Autodesk Inventor part; units mm, degrees
ref_plane "YZ Plane" through (0, 0, 0) normal (1, 0, 0) x (0, 1, 0)
ref_plane "XZ Plane" through (0, 0, 0) normal (0, 1, 0) x (-1, 0, 0)
ref_plane "XY Plane" through (0, 0, 0) normal (0, 0, 1) x (1, 0, 0)
ref_plane "Work Plane3" through (-98.2192, 25.6748, -72.651) normal (0, 1, 0) x (1, 0, 0)
sketch "Sketch1" plane through (-98.2192, 25.6748, -72.651) normal (0, 1, 0) x (1, 0, 0)
  line L0 (108.2722, -112.7231) -> (109.1382, -112.2231) construction
  line L1 (108.6382, -111.3571) -> (109.1382, -112.2231) construction
  line L2 (101.5917, -99.1522) -> (114.8917, -122.1885)
  line L3 (114.8917, -122.1885) -> (108.6563, -125.7885)
  line L4 (108.6563, -125.7885) -> (109.9613, -128.0488)
  line L5 (109.9613, -128.0488) -> (107.3632, -129.5488)
  line L6 (107.3632, -129.5488) -> (106.3632, -127.8168)
  line L7 (106.3632, -127.8168) -> (98.8635, -132.1468)
  line L8 (98.8635, -132.1468) -> (103.1935, -139.6466)
  line L9 (79.4712, -121.2385) -> (82.4842, -126.4571) construction
  line L10 (103.1935, -139.6466) -> (98.8633, -142.1466)
  line L11 (83.0235, -104.7111) -> (90.5232, -100.3811)
  line L12 (90.5232, -100.3811) -> (88.3182, -96.5619)
  line L13 (88.3182, -96.5619) -> (90.8427, -95.1044)
  line L14 (83.0235, -104.7111) -> (78.6935, -97.2113)
  line L15 (73.6327, -111.1259) -> (88.2377, -136.4225)
  line L16 (78.6935, -97.2113) -> (74.3633, -99.7113)
  line L17 (90.8427, -95.1044) -> (85.0892, -72.651)
  line L18 (104.7842, -84.0219) -> (98.2192, -72.651)
  line L19 (98.2192, -72.651) -> (85.0892, -72.651)
  line L20 (88.2377, -136.4225) -> (98.8633, -142.1466)
  line L21 (74.3633, -99.7113) -> (73.6327, -111.1259)
  line L22 (98.2192, -72.651) -> (104.7842, -84.0219)
  line L23 (104.7842, -84.0219) -> (101.5917, -99.1522)
  dimension "d1" = 26.6
  dimension "d4" = 7.2
  dimension "d5" = 2.61
  dimension "d6" = 3
  dimension "d7" = 2
  dimension "d8" = 8.66
  dimension "d9" = 8.66
  dimension "d10" = 5
  dimension "d11" = 8.66
  dimension "d12" = 31.68
  dimension "d13" = 4.41
  dimension "d14" = 2.915
  dimension "d17" = 8.66
  dimension "d18" = 29.21
  dimension "d20" = 10.27
  dimension "d21" = 5
  dimension "d22" = 23.1789
  dimension "d23" = 13.13
  dimension "d31" = 13.13
extrude "Extrusion1" add sketch "Sketch1" along normal blind 8.66
pattern_circular "Circular Pattern2" count 3 over 360 about axis through (0, 25.6748, 0) along (0, 1, 0) of "Extrusion1"
sketch "Sketch2" plane through (-98.2192, 34.3348, -72.651) normal (0, 1, 0) x (1, 0, 0)
  line L0 (46.9822, -62.321) -> (73.5822, -62.321)
  line L1 (114.8917, -122.1885) -> (101.5917, -99.1522)
  circle A0 centre (98.2192, -72.651) radius 1.5
  line L2 (98.2192, -72.651) -> (104.7842, -84.0219) construction
  line L3 (98.2192, -72.651) -> (85.0892, -72.651) construction
  line L4 (98.2192, -72.651) -> (104.7842, -61.28) construction
  circle A1 centre (98.2192, -72.651) radius 7 construction
  circle A2 centre (101.7192, -78.7131) radius 1.5
  circle A3 centre (101.7192, -66.5888) radius 1.5
  circle A4 centre (91.2192, -72.651) radius 1.5
  dimension "d35" = 3
  dimension "d36" = 14
  dimension "d37" = 3
  dimension "d38" = 3
  dimension "d39" = 3
extrude "Extrusion2" cut sketch "Sketch2" against normal blind 10
The listing builds one solid part. Answer for the finished solid, in the listing's coordinates (mm). A direction names the side the tool comes from. Round coordinates to 2 decimals unless told otherwise and drop trailing zeros. Loops run counter-clockwise (first coordinate to the right, second up) from the corner with the lowest first, then second, coordinate; pieces in that order, holes last. Notation, with made-up numbers: (81.5, 39.25) - (128.5, 39.25) arc R22 cw to (128.5, 59.25) - close; hole circle Ø6 at (-27, 17.25). An arc over 180 degrees is marked (long way). Use one line per item in the form item = value. Start each with the question number.
1. The part is cut by section C-C on y = 32.75. Give the number of separate pieces and of enclosed holes in the cut face, then the cut area to 3 significant figures.
2. A tool of negligible diameter and unlimited length cuts with its end or side. For faces 1 (the face through (-16.2, 29.944, -37.316)), 2 (the face through (-8.78, 29.94, 25.85)), 3 (the face through (-2, 34.335, -1)), 4 (the face through (-38, 30, -10.33)), from which of +Z, -Z, +X, -X, +Y, -Y can it reach the whole face along a straight path? Write none if from no direction.
3. Consider line 1 (Z direction, x = -20, y = 26.5); line 2 (X direction, y = 29.75, z = 0); line 3 (Z direction, x = -15, y = 28.75). Determine where each line is inside the solid, lowest interval first. Write a range as [from, to].
4. The part is cut by section A-A on x = -45. Determine the outline of the cut face in (y, z).
5. The part is cut by section B-B on z = 45. Determine the outline of the cut face in (x, y), then the cut area to 3 significant figures.
6. Given pin 1 Ø3 at (y, z) = (31.5, -21.5) entering from -X; pin 2 Ø4 at (y, z) = (32.5, 31) entering from -X; pin 3 Ø3 at (y, z) = (28.5, -7) entering from +X; pin 4 Ø4 at (x, z) = (0, 0) entering from +Y, each flat-ended and moving along its own axis, determine where each tip first touches the part or whether it passes through.
7. For a pull along X with two mould halves and no side action, classify faces 5 (the face through (-1.5, 30.07, -0.07)), 6 (the face through (13.6, 29.94, 51.31)), 7 (the face through (-10.213, 29.944, 11.384)) as pulls with the +X half, pulls with the -X half, needs draft (parallel to the pull), parting line crosses it, or undercut.
Geometry check:
q1.separate_pieces = 1
q1.enclosed_holes = 4
q1.area = 4,340 mm^2
q2.face_1 = -Z, +Y, -Y
q2.face_2 = +Y, -Y
q2.face_3 = +Z, -Z, +X, -X, +Y
q2.face_4 = +Z, -X, +Y, -Y
q3.line_1 = [-39.85, -29.19], [-20.53, -6.17], [24.83, 46.42]
q3.line_2 = [-13.13, -8.5], [-5.5, -1.5], [1.5, 18.19], [33.71, 46.8]
q3.line_3 = [-36.52, -29.19], [-17.4, -1.68], [31.95, 55.08]
q4.outline = (25.67, -40.53) - (34.33, -40.53) - (34.33, -10.33) - (25.67, -10.33) - close
q5.outline = (-20.82, 25.67) - (14.05, 25.67) - (14.05, 34.33) - (-20.82, 34.33) - close
q5.area = 302 mm^2
q6.pin_1 = -53.85
q6.pin_2 = -24.24
q6.pin_3 = 51.71
q6.pin_4 = 34.33
q7.face_5 = undercut
q7.face_6 = pulls with the +X half
q7.face_7 = pulls with the -X half
